Autodesk Inventor part; units mm, degrees
ref_plane "YZ Plane" through (0, 0, 0) normal (1, 0, 0) x (0, 1, 0)
ref_plane "XZ Plane" through (0, 0, 0) normal (0, 1, 0) x (-1, 0, 0)
ref_plane "XY Plane" through (0, 0, 0) normal (0, 0, 1) x (1, 0, 0)
sketch "草圖1" plane through (0, 0, 0) normal (0, 1, 0) x (-1, 0, 0)
  point P0 (0, 0)
sketch "草圖2" plane through (0, 0, 0) normal (0, 1, 0) x (-1, 0, 0)
  line L0 (0, 0) -> (100, 0)
  line L1 (100, 0) -> (100, -80)
  line L2 (100, -80) -> (0, -80)
  line L3 (0, -80) -> (0, 0)
  dimension "d0" = 100
  dimension "d1" = 80
extrude "擠出1" add sketch "草圖2" along normal blind 80
sketch "草圖3" plane through (0, 80, 0) normal (0, 1, 0) x (1, 0, 0)
  line L0 (-5, 5) -> (-95, 5)
  line L1 (-95, 5) -> (-95, 75)
  line L2 (-95, 75) -> (-5, 75)
  line L3 (-5, 75) -> (-5, 5)
  line L4 (-100, 80) -> (-100, 0)
  line L5 (0, 0) -> (0, 80)
  line L6 (-100, 0) -> (0, 0)
  line L7 (0, 80) -> (-100, 80)
  point P0 (-50, 75)
  dimension "d4" = 5
  dimension "d5" = 5
  dimension "d6" = 5
  dimension "d7" = 5
extrude "擠出2" cut sketch "草圖3" against normal blind 75 contours L0 L1 L2 L3
properties part number "MoneyCase"
CAD build for the part. Positions are in the model's coordinates, mm. A direction names the side the tool comes from. Give positions to 0.01 mm unless a question says otherwise; leave off trailing zeros. Order: outer loops, then holes, each group sorted by start corner. A loop starts at its lowest first (then second) coordinate and runs counter-clockwise, first axis right, second up.
(1) Saw through at A-A, the plane y = 44.5. Give the cut face in (x, z), then the cut area to 3 significant figures.
(2) Flat gauge pin, fed straight in: pin 1 (8 mm diameter, centred on x = -43, z = -67, fed in from +Y). Where does the tip first touch, or does it go through?
(3) Mould opens along X. For faces 1 (the flat face through (-100, 39, -39)), 2 (the flat face through (-49, 0, -39)), 3 (the flat face through (-51, 43, -75)) say: released by +X, released by -X, zero draft, split by the parting line, or undercut.
(4) Saw through at C-C, the plane z = -31. Give the cut face in (x, y), then the cut area to 3 significant figures.
(5) Saw through at B-B, the plane x = -10.5. Give the cut face in (y, z), then the cut area to 3 significant figures.
(6) Drill centre lines: L1, parallel to Z at x = -67, y = 41; L2, parallel to X at y = 68, z = -17.5; L3, parallel to Y at x = -44.5, z = -62. Where is each one in solid material? Low to high.
(7) Tool access for faces 4 (the flat face through (0, 39, -41)), 5 (the flat face through (-5, 43, -40)): list every direction of +Z, -Z, +X, -X, +Y, -Y with a clear straight run to the whole face (end or side of a thin tool).
Results found:
1. outline: (-100, -80) - (0, -80) - (0, 0) - (-100, 0) - close; hole (-95, -75) - (-5, -75) - (-5, -5) - (-95, -5) - close
1. area: 1,700 mm2
2. pin 1: stops at y = 5
3. face 1: released by -X
3. face 2: zero draft
3. face 3: undercut
4. outline: (-100, 0) - (0, 0) - (0, 80) - (-5, 80) - (-5, 5) - (-95, 5) - (-95, 80) - (-100, 80) - close
4. area: 1,250 mm2
5. outline: (0, -80) - (80, -80) - (80, -75) - (5, -75) - (5, -5) - (80, -5) - (80, 0) - (0, 0) - close
5. area: 1,150 mm2
6. L1: z = -80 to -75, -5 to 0
6. L2: x = -100 to -95, -5 to 0
6. L3: y = 0 to 5
7. face 4: +Z, -Z, +X, +Y, -Y
7. face 5: +Y
